```python
from build123d import *

# Parameters (mm, degrees)
F0_W     = 15
F0_H     = 8
F1_DEPTH = 24
F2_W     = 8
F2_H     = 16
F3_DEPTH = 19.8
F4_W     = 20
F4_H     = 8
F5_DEPTH = 8


with BuildPart() as f1:
    # F0 (on Top) → F1 (new body)
    with BuildSketch(Plane.XY):
        with Locations((7.5, 4)):
            Rectangle(F0_W, F0_H)
    extrude(amount=F1_DEPTH)

    # F2 (on face) → F3 (join)
    with BuildSketch(Plane.YZ.offset(15)):
        with Locations((4, 8)):
            Rectangle(F2_W, F2_H)
    extrude(amount=F3_DEPTH)

    # F4 (on Top) → F5 (join)
    with BuildSketch(Plane.XY):
        with Locations((10, -4)):
            Rectangle(F4_W, F4_H)
    extrude(amount=F5_DEPTH)


solid = f1.part
```
Could you check a few things on this model? Use its own coordinates, in mm. A direction names the side the tool comes from. Coordinates: 2 decimals unless noted, no trailing zeros. Loops run counter-clockwise (first coordinate to the right, second up) from the corner with the lowest first, then second, coordinate; pieces in that order, holes last.
1) Which directions (+Z, -Z, +X, -X, +Y, -Y) give clear straight access to the entire face, cutting with the end or side of a thin tool? Please do faces 1 (the face through (10, -4, 8)), 2 (the face through (7, 4, 24)), 3 (the face through (20, -4, 4)), 4 (the face through (15, 4, 20)).
Reported:
face 1: +Z, +X, -X, -Y
face 2: +Z, +X, -X, +Y, -Y
face 3: +Z, -Z, +X, -Y
face 4: +Z, +X, +Y, -Y
2) Please list where these lines run through material, in increasing order: line 1 along Y through (x, z) = (4.5, 20.5); line 2 along X through (y, z) = (2.75, 21.25); line 3 along Z through (x, y) = (18, 2.75).
Reported:
line 1: y = 0 to 8
line 2: x = 0 to 15
line 3: z = 0 to 16
3) Imagine slicing it at B-B (z = 3). List the corners of the cut face in (x, y) for me, and give its area (3 significant figures).
Reported:
outline: (0, -8) - (20, -8) - (20, 0) - (34.8, 0) - (34.8, 8) - (0, 8) - close
area: 438 mm2
4) Imagine slicing it at C-C (x = 24). List the corners of the cut face in (y, z) for me.
Reported:
outline: (0, 0) - (8, 0) - (8, 16) - (0, 16) - close
5) Imagine slicing it at A-A (y = 4.5). List the corners of the cut face in (x, z) for me.
Reported:
outline: (0, 0) - (34.8, 0) - (34.8, 16) - (15, 16) - (15, 24) - (0, 24) - close
6) Imagine slicing it at D-D (z = 9.5). List the corners of the cut face in (x, y) for me, and give its area (3 significant figures).
Reported:
outline: (0, 0) - (34.8, 0) - (34.8, 8) - (0, 8) - close
area: 278 mm2
7) Will these pins go through, and if not, where does the flat tip stop? pin 1 Ø6.5 at (y, z) = (-4.5, 3) entering from +X; pin 2 Ø3 at (y, z) = (-1, 17.5) entering from +X; pin 3 Ø6.5 at (x, y) = (12, -2.5) entering from +Z; pin 4 Ø4 at (x, z) = (26.5, 16.5) entering from -Y.
Reported:
pin 1: stops at x = 20
pin 2: stops at x = 15
pin 3: stops at z = 24
pin 4: stops at y = 0
